CAD build for the part. Positions are in the model's coordinates, mm. Face numbers are marked on the shaded views. Give positions to 0.01 mm unless a question says otherwise; leave off trailing zeros. Order: outer loops, then holes, each group sorted by start corner. A loop starts at its lowest first (then second) coordinate and runs counter-clockwise, first axis right, second up. Notation, with made-up numbers: M 53.5,40.5 L 61.5,40.5 A6 cw 61.5,49.5 Z; hole C -7.5,32.5 d7. An arc over 180 degrees is marked long. Put each result on its own line as item: value. Start each with the question number.
1) Two-plate mould, pull along Z, no slides. Class the marked faces 1, 2 and 3: released by +Z, released by -Z, zero draft, split by the parting line, or undercut.
2) Cut at B-B (z = -232.5). Write the cut outline in (x, y), and give its area (3 significant figures).
3) Pin check, flat tips, straight feed: pin 1 (3 mm diameter, centred on x = -102.5, y = -26.5, fed in from +Z); pin 2 (22.5 mm diameter, centred on x = -50, z = -291.5, fed in from -Y); pin 3 (6 mm diameter, centred on x = 200, y = -50, fed in from -Z); pin 4 (13 mm diameter, centred on x = -200, y = -50, fed in from +Z). Stop position of each tip, or through.
4) Cut at C-C (y = -130). Write the cut outline in (x, z).
5) Cut at A-A (x = -10.5). Write the cut outline in (y, z).
6) Drill centre lines: line 1 (Z direction, x = 229, y = -30); line 2 (Z direction, x = -44, y = 4.5); line 3 (X direction, y = -50, z = -201.5). Where is each one in solid material? Low to high. Write a range as [from, to].
```python
from build123d import *

# Parameters (mm, degrees)
BOSS_EXTRUDE1_START = 300
SKETCH1_R           = 25
SKETCH1_R_2         = 15
SKETCH1_R_3         = 5
BOSS_EXTRUDE1_DEPTH = 28
BOSS_EXTRUDE2_DEPTH = 300
BOSS_EXTRUDE3_START = 170
BOSS_EXTRUDE3_DEPTH = 100
BOSS_EXTRUDE4_START = 137
SKETCH1_6_R         = 25
SKETCH1_6_R_2       = 15
BOSS_EXTRUDE4_DEPTH = 28


with BuildPart() as part:
    # Sketch1 → Boss-Extrude1 (new body)
    # profile 1 of 8: a face of its own
    with BuildSketch(Plane.XY.offset(BOSS_EXTRUDE1_START)):
        with BuildLine():
            Line((-272, 0), (-114.644660941, 0))
            Line((-114.644660941, 0), (-113.397459622, 0))
            ThreePointArc((-113.397459622, 0), (-124.107281107, 15.11754924), (-137.422048611, 28))
            Line((-137.422048611, 28), (-262.577951389, 28))
            ThreePointArc((-262.577951389, 28), (-267.426310923, 23.849120478), (-272, 19.397406292))
            Line((-272, 19.397406292), (-272, 0))
        make_face()
    # profile 2 of 8: a face of its own
    with BuildSketch(Plane.XY.offset(BOSS_EXTRUDE1_START)):
        with BuildLine():
            Line((-272, 28), (-272, 19.397406292))
            ThreePointArc((-272, 19.397406292), (-267.426310923, 23.849120478), (-262.577951389, 28))
            Line((-262.577951389, 28), (-272, 28))
        make_face()
    # profile 3 of 8: a face of its own
    with BuildSketch(Plane.XY.offset(BOSS_EXTRUDE1_START)):
        with BuildLine():
            Line((-285.355339059, 0), (-272, 0))
            Line((-272, 0), (-272, 19.397406292))
            ThreePointArc((-272, 19.397406292), (-279.89215416, 10.143525867), (-286.602540378, 0))
            Line((-286.602540378, 0), (-285.355339059, 0))
        make_face()
    # profile 4 of 8: a face of its own
    with BuildSketch(Plane.XY.offset(BOSS_EXTRUDE1_START)):
        with BuildLine():
            ThreePointArc((-137.422048611, 28), (-124.107281107, 15.11754924), (-113.397459622, 0))
            Line((-113.397459622, 0), (0, 0))
            Line((0, 0), (0, 28))
            Line((0, 28), (-137.422048611, 28))
        make_face()
    # profile 5 of 8: a face of its own
    with BuildSketch(Plane.XY.offset(BOSS_EXTRUDE1_START)):
        with BuildLine():
            ThreePointArc((-286.602540378, 0), (-279.89215416, 10.143525867), (-272, 19.397406292))
            Line((-272, 19.397406292), (-272, 28))
            Line((-272, 28), (-300, 28))
            Line((-300, 28), (-300, 0))
            Line((-300, 0), (-286.602540378, 0))
        make_face()
    # profile 6 of 8: a face of its own
    with BuildSketch(Plane.XY.offset(BOSS_EXTRUDE1_START)):
        with BuildLine():
            Line((-182.32233047, -67.67766953), (-114.644660941, 0))
            Line((-114.644660941, 0), (-272, 0))
            Line((-272, 0), (-285.355339059, 0))
            Line((-285.355339059, 0), (-217.67766953, -67.67766953))
            ThreePointArc((-217.67766953, -67.67766953), (-209.567085809, -26.903011687), (-175, -50))
            ThreePointArc((-175, -50), (-176.903011687, -59.567085809), (-182.32233047, -67.67766953))
        make_face()
    # profile 7 of 8: a face of its own
    with BuildSketch(Plane.XY.offset(BOSS_EXTRUDE1_START)):
        with Locations((-200, -50)):
            Circle(SKETCH1_R)
        with Locations((-200, -50)):
            Circle(SKETCH1_R_2, mode=Mode.SUBTRACT)
    # profile 8 of 8: a face of its own
    with BuildSketch(Plane.XY.offset(BOSS_EXTRUDE1_START)):
        with Locations((-200, -50)):
            Circle(SKETCH1_R_2)
        with Locations((-200, -50)):
            Circle(SKETCH1_R_3, mode=Mode.SUBTRACT)
    extrude(amount=-BOSS_EXTRUDE1_DEPTH)

    # Sketch1_4 → Boss-Extrude2 (add)
    with BuildSketch(Plane.XY):
        with BuildLine():
            ThreePointArc((-286.602540378, 0), (-279.89215416, 10.143525867), (-272, 19.397406292))
            Line((-272, 19.397406292), (-272, 28))
            Line((-272, 28), (-300, 28))
            Line((-300, 28), (-300, 0))
            Line((-300, 0), (-286.602540378, 0))
        make_face()
    extrude(amount=BOSS_EXTRUDE2_DEPTH)

    # Sketch1_5 → Boss-Extrude3 (add)
    with BuildSketch(Plane.XY.offset(BOSS_EXTRUDE3_START)):
        with BuildLine():
            Line((-262.577951389, 28), (-137.422048611, 28))
            ThreePointArc((-137.422048611, 28), (-200, 50), (-262.577951389, 28))
        make_face()
        with BuildLine():
            Line((-272, 0), (-114.644660941, 0))
            Line((-114.644660941, 0), (-113.397459622, 0))
            ThreePointArc((-113.397459622, 0), (-124.107281107, 15.11754924), (-137.422048611, 28))
            Line((-137.422048611, 28), (-262.577951389, 28))
            ThreePointArc((-262.577951389, 28), (-267.426310923, 23.849120478), (-272, 19.397406292))
            Line((-272, 19.397406292), (-272, 0))
        make_face()
        with BuildLine():
            Line((-182.32233047, -67.67766953), (-114.644660941, 0))
            Line((-114.644660941, 0), (-272, 0))
            Line((-272, 0), (-285.355339059, 0))
            Line((-285.355339059, 0), (-217.67766953, -67.67766953))
            ThreePointArc((-217.67766953, -67.67766953), (-209.567085809, -26.903011687), (-175, -50))
            ThreePointArc((-175, -50), (-176.903011687, -59.567085809), (-182.32233047, -67.67766953))
        make_face()
        with BuildLine():
            Line((-113.397459622, 0), (-114.644660941, 0))
            Line((-114.644660941, 0), (-182.32233047, -67.67766953))
            ThreePointArc((-182.32233047, -67.67766953), (-200, -75), (-217.67766953, -67.67766953))
            Line((-217.67766953, -67.67766953), (-285.355339059, 0))
            Line((-285.355339059, 0), (-286.602540378, 0))
            ThreePointArc((-286.602540378, 0), (-225.88190451, -146.592582629), (-100, -50))
            ThreePointArc((-100, -50), (-103.407417371, -24.11809549), (-113.397459622, 0))
        make_face()
        with BuildLine():
            Line((-285.355339059, 0), (-272, 0))
            Line((-272, 0), (-272, 19.397406292))
            ThreePointArc((-272, 19.397406292), (-279.89215416, 10.143525867), (-286.602540378, 0))
            Line((-286.602540378, 0), (-285.355339059, 0))
        make_face()
    extrude(amount=BOSS_EXTRUDE3_DEPTH)

    # Sketch1_6 → Boss-Extrude4 (add)
    # profile 1 of 7: a face of its own
    with BuildSketch(Plane.XY.offset(BOSS_EXTRUDE4_START)):
        with BuildLine():
            ThreePointArc((-137.422048611, 28), (-124.107281107, 15.11754924), (-113.397459622, 0))
            Line((-113.397459622, 0), (0, 0))
            Line((0, 0), (0, 28))
            Line((0, 28), (-137.422048611, 28))
        make_face()
    # profile 2 of 7: a face of its own
    with BuildSketch(Plane.XY.offset(BOSS_EXTRUDE4_START)):
        with BuildLine():
            Line((-272, 0), (-114.644660941, 0))
            Line((-114.644660941, 0), (-113.397459622, 0))
            ThreePointArc((-113.397459622, 0), (-124.107281107, 15.11754924), (-137.422048611, 28))
            Line((-137.422048611, 28), (-262.577951389, 28))
            ThreePointArc((-262.577951389, 28), (-267.426310923, 23.849120478), (-272, 19.397406292))
            Line((-272, 19.397406292), (-272, 0))
        make_face()
    # profile 3 of 7: a face of its own
    with BuildSketch(Plane.XY.offset(BOSS_EXTRUDE4_START)):
        with BuildLine():
            Line((-182.32233047, -67.67766953), (-114.644660941, 0))
            Line((-114.644660941, 0), (-272, 0))
            Line((-272, 0), (-285.355339059, 0))
            Line((-285.355339059, 0), (-217.67766953, -67.67766953))
            ThreePointArc((-217.67766953, -67.67766953), (-209.567085809, -26.903011687), (-175, -50))
            ThreePointArc((-175, -50), (-176.903011687, -59.567085809), (-182.32233047, -67.67766953))
        make_face()
    # profile 4 of 7: a face of its own
    with BuildSketch(Plane.XY.offset(BOSS_EXTRUDE4_START)):
        with Locations((-200, -50)):
            Circle(SKETCH1_6_R)
        with Locations((-200, -50)):
            Circle(SKETCH1_6_R_2, mode=Mode.SUBTRACT)
    # profile 5 of 7: a face of its own
    with BuildSketch(Plane.XY.offset(BOSS_EXTRUDE4_START)):
        with BuildLine():
            Line((-272, 28), (-272, 19.397406292))
            ThreePointArc((-272, 19.397406292), (-267.426310923, 23.849120478), (-262.577951389, 28))
            Line((-262.577951389, 28), (-272, 28))
        make_face()
    # profile 6 of 7: a face of its own
    with BuildSketch(Plane.XY.offset(BOSS_EXTRUDE4_START)):
        with BuildLine():
            ThreePointArc((-286.602540378, 0), (-279.89215416, 10.143525867), (-272, 19.397406292))
            Line((-272, 19.397406292), (-272, 28))
            Line((-272, 28), (-300, 28))
            Line((-300, 28), (-300, 0))
            Line((-300, 0), (-286.602540378, 0))
        make_face()
    # profile 7 of 7: a face of its own
    with BuildSketch(Plane.XY.offset(BOSS_EXTRUDE4_START)):
        with BuildLine():
            Line((-285.355339059, 0), (-272, 0))
            Line((-272, 0), (-272, 19.397406292))
            ThreePointArc((-272, 19.397406292), (-279.89215416, 10.143525867), (-286.602540378, 0))
            Line((-286.602540378, 0), (-285.355339059, 0))
        make_face()
    extrude(amount=BOSS_EXTRUDE4_DEPTH)

    # Mirror1: part across plane


with BuildPart() as part_1:
    add(part.part)
    add(part.part.mirror(Plane.XY))

    # Mirror2: part across plane


with BuildPart() as part_2:
    add(part_1.part)
    add(part_1.part.mirror(Plane(origin=(0, 0, 0), x_dir=(0, 0, 1), z_dir=(1, 0, 0))))


solid = part_2.part
```
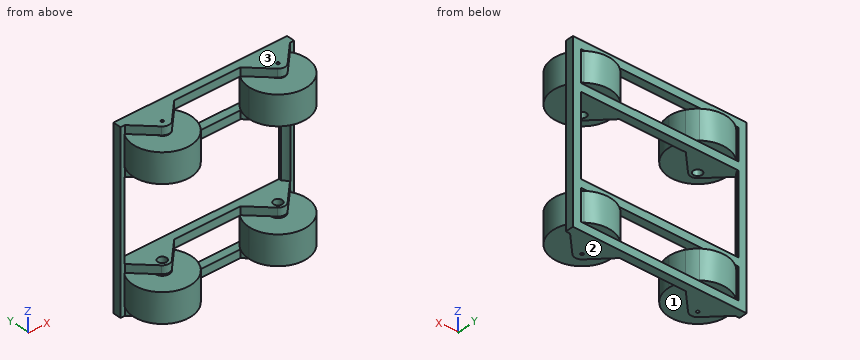
Solution:
1. face 1: undercut
1. face 2: released by -Z
1. face 3: released by +Z
2. outline: M -300,0 L -286.6,0 A100 ccw long -272,19.4 L -272,28 L -300,28 Z; M 272,19.4 A100 ccw long 286.6,0 L 300,0 L 300,28 L 272,28 Z; hole C -200,-50 d50; hole C 200,-50 d50
2. area: 60,200 mm²
3. pin 1: z = 270
3. pin 2: y = 0
3. pin 3: through
3. pin 4: z = 300
4. outline: M -260,-270 L -140,-270 L -140,-170 L -260,-170 Z; M -260,170 L -140,170 L -140,270 L -260,270 Z; M 140,-270 L 260,-270 L 260,-170 L 140,-170 Z; M 140,170 L 260,170 L 260,270 L 140,270 Z
5. outline: M 0,-300 L 28,-300 L 28,-272 L 0,-272 Z; M 0,-165 L 28,-165 L 28,-137 L 0,-137 Z; M 0,137 L 28,137 L 28,165 L 0,165 Z; M 0,272 L 28,272 L 28,300 L 0,300 Z
6. line 1: [-300, -272], [-270, -170], [-165, -137], [137, 165], [170, 270], [272, 300]
6. line 2: [-300, -272], [-165, -137], [137, 165], [272, 300]
6. line 3: [-300, -225], [-175, -100], [100, 175], [225, 300]
